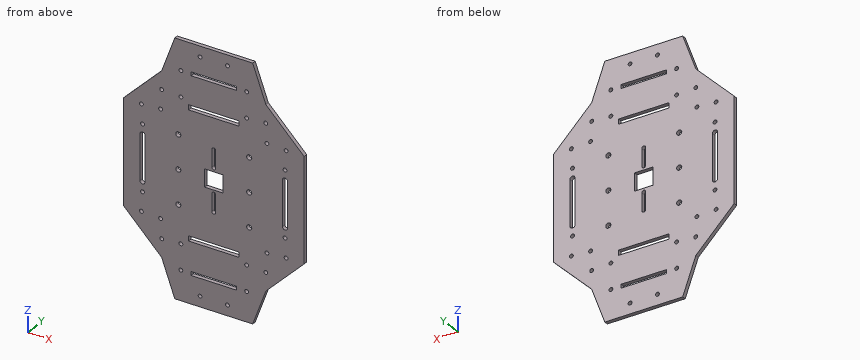
```python
from build123d import *

# Parameters (mm, degrees)
SKETCH_1_W                                 = 141.421356238
SKETCH_1_H                                 = 141.421356238
EXTRUDE_1_DEPTH                            = 3
CUT_EXTRUDE_1_DEPTH                        = 3
MIRROR_1_AT_THE_SECOND_PLANE_COPY_1_DEPTH  = 3
SKETCH_3_R                                 = 1.5
CUT_EXTRUDE_2_DEPTH                        = 3
MIRROR_2_AT_THE_SECOND_PLANE_COPY_1_SKET_R = 1.5
MIRROR_2_AT_THE_SECOND_PLANE_COPY_1_DEPTH  = 3
SKETCH_4_R                                 = 2
CUT_EXTRUDE_3_DEPTH                        = 3
SKETCH_5_R                                 = 1.5
CUT_EXTRUDE_4_DEPTH                        = 3
MIRROR_4_AT_THE_SECOND_PLANE_COPY_1_SKET_R = 1.5
MIRROR_4_AT_THE_SECOND_PLANE_COPY_1_DEPTH  = 3
SKETCH_6_R                                 = 1.5
CUT_EXTRUDE_5_DEPTH                        = 3
MIRROR_5_AT_THE_SECOND_PLANE_COPY_1_SKET_R = 1.5
MIRROR_5_AT_THE_SECOND_PLANE_COPY_1_DEPTH  = 3
CUT_EXTRUDE_6_DEPTH                        = 3
SKETCH_8_W                                 = 14.436516826
SKETCH_8_H                                 = 13.841494932
CUT_EXTRUDE_7_DEPTH                        = 3
CUT_EXTRUDE_8_DEPTH                        = 3
CUT_EXTRUDE_10_DEPTH                       = 3
EXTRUDE_2_DEPTH                            = 3
MIRROR_9_AT_THE_SECOND_PLANE_COPY_1_DEPTH  = 3
SKETCH_13_R                                = 1.5
CUT_EXTRUDE_11_DEPTH                       = 3
MIRROR_11_COPY_1_SKETCH_R                  = 1.5
MIRROR_11_COPY_1_DEPTH                     = 3


with BuildPart() as part:
    # 草图1 → 凸台-拉伸1 (new body)
    with BuildSketch(Plane(origin=(0, 0, 0), x_dir=(1, 0, 0), z_dir=(0, 1, 0))):
        Rectangle(SKETCH_1_W, SKETCH_1_H)
    extrude(amount=EXTRUDE_1_DEPTH)

    # 草图2 → 切除-拉伸1 (cut)
    with BuildSketch(Plane(origin=(0, 0, 0), x_dir=(1, 0, 0), z_dir=(0, 1, 0))):
        Polygon((-70.710678119, 70.710678119), (-40.710678119, 70.710678119), (-70.710678119, 40.710678119), align=None)
    cut_extrude_1 = extrude(amount=CUT_EXTRUDE_1_DEPTH, mode=Mode.SUBTRACT)

    # 镜向1: 切除-拉伸1 across plane
    add(cut_extrude_1.mirror(Plane(origin=(0, 0, 0), x_dir=(0, 0, 1), z_dir=(1, 0, 0))), mode=Mode.SUBTRACT)

    # 镜向1 at the second plane: 切除-拉伸1 across plane
    add(cut_extrude_1.mirror(Plane.XY), mode=Mode.SUBTRACT)

    # 镜向1 at the second plane copy 1 sket → 镜向1 at the second plane copy 1 (cut)
    with BuildSketch(Plane(origin=(0, 0, 0), x_dir=(-1, 0, 0), z_dir=(0, 1, 0))):
        Polygon((-70.710678119, 70.710678119), (-40.710678119, 70.710678119), (-70.710678119, 40.710678119), align=None)
    extrude(amount=MIRROR_1_AT_THE_SECOND_PLANE_COPY_1_DEPTH, mode=Mode.SUBTRACT)

    # 草图3 → 切除-拉伸2 (cut)
    with BuildSketch(Plane(origin=(0, 0, 0), x_dir=(1, 0, 0), z_dir=(0, 1, 0))):
        with Locations(Location((-56.568542495, 40.710678119, 0), (0, 0, 270))):
            Circle(SKETCH_3_R)
        with Locations(Location((-40.710678119, 56.568542495, 0), (0, 0, 270))):
            Circle(SKETCH_3_R)
        with Locations(Location((-41.568542495, 41.568542495, 0), (0, 0, 270))):
            Circle(SKETCH_3_R)
    cut_extrude_2 = extrude(amount=CUT_EXTRUDE_2_DEPTH, mode=Mode.SUBTRACT)

    # 镜向2: 切除-拉伸2 across plane
    add(cut_extrude_2.mirror(Plane.XY), mode=Mode.SUBTRACT)

    # 镜向2 at the second plane: 切除-拉伸2 across plane
    add(cut_extrude_2.mirror(Plane(origin=(0, 0, 0), x_dir=(0, 0, 1), z_dir=(1, 0, 0))), mode=Mode.SUBTRACT)

    # 镜向2 at the second plane copy 1 sket → 镜向2 at the second plane copy 1 (cut)
    with BuildSketch(Plane(origin=(0, 0, 0), x_dir=(-1, 0, 0), z_dir=(0, 1, 0))):
        with Locations(Location((-56.568542495, 40.710678119, 0), (0, 0, 270))):
            Circle(MIRROR_2_AT_THE_SECOND_PLANE_COPY_1_SKET_R)
        with Locations(Location((-40.710678119, 56.568542495, 0), (0, 0, 270))):
            Circle(MIRROR_2_AT_THE_SECOND_PLANE_COPY_1_SKET_R)
        with Locations(Location((-41.568542495, 41.568542495, 0), (0, 0, 270))):
            Circle(MIRROR_2_AT_THE_SECOND_PLANE_COPY_1_SKET_R)
    extrude(amount=MIRROR_2_AT_THE_SECOND_PLANE_COPY_1_DEPTH, mode=Mode.SUBTRACT)

    # 草图4 → 切除-拉伸3 (cut)
    with BuildSketch(Plane(origin=(0, 0, 0), x_dir=(1, 0, 0), z_dir=(0, 1, 0))):
        with Locations(Location((-27.710678119, 26.568542495, 0), (0, 0, 270))):
            Circle(SKETCH_4_R)
        with Locations(Location((-27.710678119, -26.568542495, 0), (0, 0, 270))):
            Circle(SKETCH_4_R)
        with Locations(Location((-27.710678119, 0, 0), (0, 0, 270))):
            Circle(SKETCH_4_R)
    cut_extrude_3 = extrude(amount=CUT_EXTRUDE_3_DEPTH, mode=Mode.SUBTRACT)

    # 镜向3: 切除-拉伸3 across plane
    add(cut_extrude_3.mirror(Plane(origin=(0, 0, 0), x_dir=(0, 0, 1), z_dir=(1, 0, 0))), mode=Mode.SUBTRACT)

    # 草图5 → 切除-拉伸4 (cut)
    with BuildSketch(Plane(origin=(0, 0, 0), x_dir=(1, 0, 0), z_dir=(0, 1, 0))):
        with Locations(Location((-55.710678119, 25.710678119, 0), (0, 0, 270))):
            Circle(SKETCH_5_R)
    cut_extrude_4 = extrude(amount=CUT_EXTRUDE_4_DEPTH, mode=Mode.SUBTRACT)

    # 镜向4: 切除-拉伸4 across plane
    add(cut_extrude_4.mirror(Plane(origin=(0, 0, 0), x_dir=(0, 0, 1), z_dir=(1, 0, 0))), mode=Mode.SUBTRACT)

    # 镜向4 at the second plane: 切除-拉伸4 across plane
    add(cut_extrude_4.mirror(Plane.XY), mode=Mode.SUBTRACT)

    # 镜向4 at the second plane copy 1 sket → 镜向4 at the second plane copy 1 (cut)
    with BuildSketch(Plane(origin=(0, 0, 0), x_dir=(-1, 0, 0), z_dir=(0, 1, 0))):
        with Locations(Location((-55.710678119, 25.710678119, 0), (0, 0, 270))):
            Circle(MIRROR_4_AT_THE_SECOND_PLANE_COPY_1_SKET_R)
    extrude(amount=MIRROR_4_AT_THE_SECOND_PLANE_COPY_1_DEPTH, mode=Mode.SUBTRACT)

    # 草图6 → 切除-拉伸5 (cut)
    with BuildSketch(Plane(origin=(0, 0, 0), x_dir=(1, 0, 0), z_dir=(0, 1, 0))):
        with Locations(Location((-25.710678119, 55.710678119, 0), (0, 0, 270))):
            Circle(SKETCH_6_R)
    cut_extrude_5 = extrude(amount=CUT_EXTRUDE_5_DEPTH, mode=Mode.SUBTRACT)

    # 镜向5: 切除-拉伸5 across plane
    add(cut_extrude_5.mirror(Plane.XY), mode=Mode.SUBTRACT)

    # 镜向5 at the second plane: 切除-拉伸5 across plane
    add(cut_extrude_5.mirror(Plane(origin=(0, 0, 0), x_dir=(0, 0, 1), z_dir=(1, 0, 0))), mode=Mode.SUBTRACT)

    # 镜向5 at the second plane copy 1 sket → 镜向5 at the second plane copy 1 (cut)
    with BuildSketch(Plane(origin=(0, 0, 0), x_dir=(-1, 0, 0), z_dir=(0, 1, 0))):
        with Locations(Location((-25.710678119, 55.710678119, 0), (0, 0, 270))):
            Circle(MIRROR_5_AT_THE_SECOND_PLANE_COPY_1_SKET_R)
    extrude(amount=MIRROR_5_AT_THE_SECOND_PLANE_COPY_1_DEPTH, mode=Mode.SUBTRACT)

    # 草图7 → 切除-拉伸6 (cut)
    with BuildSketch(Plane(origin=(0, 0, 0), x_dir=(1, 0, 0), z_dir=(0, 1, 0))):
        with BuildLine():
            Line((-53.710678119, 17.710678119), (-53.710678119, -17.710678119))
            ThreePointArc((-53.710678119, -17.710678119), (-55.710678119, -19.710678119), (-57.710678119, -17.710678119))
            Line((-57.710678119, -17.710678119), (-57.710678119, 17.710678119))
            ThreePointArc((-57.710678119, 17.710678119), (-55.710678119, 19.710678119), (-53.710678119, 17.710678119))
        make_face()
    cut_extrude_6 = extrude(amount=CUT_EXTRUDE_6_DEPTH, mode=Mode.SUBTRACT)

    # 镜向6: 切除-拉伸6 across plane
    add(cut_extrude_6.mirror(Plane(origin=(0, 0, 0), x_dir=(0, 0, 1), z_dir=(1, 0, 0))), mode=Mode.SUBTRACT)

    # 草图8 → 切除-拉伸7 (cut)
    with BuildSketch(Plane(origin=(0, 0, 0), x_dir=(1, 0, 0), z_dir=(0, 1, 0))):
        Rectangle(SKETCH_8_W, SKETCH_8_H)
    extrude(amount=CUT_EXTRUDE_7_DEPTH, mode=Mode.SUBTRACT)

    # 草图9 → 切除-拉伸8 (cut)
    with BuildSketch(Plane(origin=(0, 0, 0), x_dir=(1, 0, 0), z_dir=(0, 1, 0))):
        with BuildLine():
            Line((1.5, -9.920747466), (1.5, -23.568542495))
            ThreePointArc((1.5, -23.568542495), (0, -25.068542495), (-1.5, -23.568542495))
            Line((-1.5, -23.568542495), (-1.5, -9.920747466))
            ThreePointArc((-1.5, -9.920747466), (0, -8.420747466), (1.5, -9.920747466))
        make_face()
    cut_extrude_8 = extrude(amount=CUT_EXTRUDE_8_DEPTH, mode=Mode.SUBTRACT)

    # 镜向7: 切除-拉伸8 across plane
    add(cut_extrude_8.mirror(Plane.XY), mode=Mode.SUBTRACT)

    # 草图10 → 切除-拉伸10 (cut)
    with BuildSketch(Plane(origin=(0, 0, 0), x_dir=(1, 0, 0), z_dir=(0, 1, 0))):
        Polygon((-19.710678119, 51.710678119), (-19.710678119, 51.490395466), (-19.710678119, 47.710678119), (19.710678119, 47.710678119), (19.710678119, 51.710678119), align=None)
    cut_extrude_10 = extrude(amount=CUT_EXTRUDE_10_DEPTH, mode=Mode.SUBTRACT)

    # 镜向8: 切除-拉伸10 across plane
    add(cut_extrude_10.mirror(Plane.XY), mode=Mode.SUBTRACT)

    # 草图11 → 凸台-拉伸2 (add)
    with BuildSketch(Plane(origin=(0, 3, 0), x_dir=(1, 0, 0), z_dir=(0, 1, 0))):
        Polygon((-40.710678119, 70.710678119), (-30.450073819, 98.901456742), (30.450073819, 98.901456742), (40.710678119, 70.710678119), align=None)
    extrude_2 = extrude(amount=-EXTRUDE_2_DEPTH)

    # 镜向9: 凸台-拉伸2 across plane
    add(extrude_2.mirror(Plane(origin=(0, 0, 0), x_dir=(0, 0, 1), z_dir=(1, 0, 0))))

    # 镜向9 at the second plane: 凸台-拉伸2 across plane
    add(extrude_2.mirror(Plane.XY))

    # 镜向9 at the second plane copy 1 sket → 镜向9 at the second plane copy 1 (add)
    with BuildSketch(Plane(origin=(0, 3, 0), x_dir=(-1, 0, 0), z_dir=(0, 1, 0))):
        Polygon((-40.710678119, 70.710678119), (-30.450073819, 98.901456742), (30.450073819, 98.901456742), (40.710678119, 70.710678119), align=None)
    extrude(amount=-MIRROR_9_AT_THE_SECOND_PLANE_COPY_1_DEPTH)

    # 草图13 → 切除-拉伸11 (cut)
    with BuildSketch(Plane.XZ):
        with Locations(Location((-25.710678119, 75.710678119, 0), (0, 0, 270))):
            Circle(SKETCH_13_R)
        with Locations(Location((-10.710678119, 90.710678119, 0), (0, 0, 270))):
            Circle(SKETCH_13_R)
        Polygon((-17.710678119, 75.710678119), (-17.710678119, 77.210678119), (0, 77.210678119), (0, 74.210678119), (-17.710678119, 74.210678119), align=None)
    cut_extrude_11 = extrude(amount=-CUT_EXTRUDE_11_DEPTH, mode=Mode.SUBTRACT)

    # 镜向10: 切除-拉伸11 across plane
    add(cut_extrude_11.mirror(Plane(origin=(0, 0, 0), x_dir=(0, 0, 1), z_dir=(1, 0, 0))), mode=Mode.SUBTRACT)

    # 镜向11: 切除-拉伸11 across plane
    add(cut_extrude_11.mirror(Plane.XY), mode=Mode.SUBTRACT)

    # 镜向11 copy 1 sketch → 镜向11 copy 1 (cut)
    with BuildSketch(Plane(origin=(0, 0, 0), x_dir=(-1, 0, 0), z_dir=(0, -1, 0))):
        with Locations(Location((-25.710678119, 75.710678119, 0), (0, 0, 270))):
            Circle(MIRROR_11_COPY_1_SKETCH_R)
        with Locations(Location((-10.710678119, 90.710678119, 0), (0, 0, 270))):
            Circle(MIRROR_11_COPY_1_SKETCH_R)
        Polygon((-17.710678119, 75.710678119), (-17.710678119, 77.210678119), (0, 77.210678119), (0, 74.210678119), (-17.710678119, 74.210678119), align=None)
    extrude(amount=-MIRROR_11_COPY_1_DEPTH, mode=Mode.SUBTRACT)


solid = part.part
```
Could you check a few things on this model? Use its own coordinates, in mm. Coordinates: 2 decimals unless noted, no trailing zeros. Loops run counter-clockwise (first coordinate to the right, second up) from the corner with the lowest first, then second, coordinate; pieces in that order, holes last.
1) Will these pins go through, and if not, where does the flat tip stop? pin 1 Ø1 at (y, z) = (1.5, -70) entering from +X; pin 2 Ø4 at (x, z) = (-10.71, -90.71) entering from -Y.
Reported:
pin 1: stops at x = 41.92
pin 2: stops at y = 0
2) Imagine slicing it at A-A (z = 0). List the corners of the cut face in (x, y) for me, and give its area (3 significant figures).
Reported:
outline: (-70.71, 0) - (-57.71, 0) - (-57.71, 3) - (-70.71, 3) - close; (-53.71, 0) - (-29.71, 0) - (-29.71, 3) - (-53.71, 3) - close; (-25.71, 0) - (-7.22, 0) - (-7.22, 3) - (-25.71, 3) - close; (7.22, 0) - (25.71, 0) - (25.71, 3) - (7.22, 3) - close; (29.71, 0) - (53.71, 0) - (53.71, 3) - (29.71, 3) - close; (57.71, 0) - (70.71, 0) - (70.71, 3) - (57.71, 3) - close
area: 333 mm2
3) Please list where these lines run through material, in increasing order: line 1 along Z through (x, y) = (17.5, 0.75); line 2 along X through (y, z) = (2.55, 13.5); line 3 along Z through (x, y) = (6.5, 1.55).
Reported:
line 1: z = -98.9 to -77.21, -74.21 to -51.71, -47.71 to 47.71, 51.71 to 74.21, 77.21 to 98.9
line 2: x = -70.71 to -57.71, -53.71 to -1.5, 1.5 to 53.71, 57.71 to 70.71
line 3: z = -98.9 to -77.21, -74.21 to -51.71, -47.71 to -6.92, 6.92 to 47.71, 51.71 to 74.21, 77.21 to 98.9
4) Imagine slicing it at C-C (x = 45.5). List the corners of the cut face in (y, z) for me.
Reported:
outline: (0, -65.92) - (3, -65.92) - (3, 65.92) - (0, 65.92) - close
5) Imagine slicing it at B-B (y = 1.25). State how many separate pieces and enclosed holes the cut face has, and give its area (3 significant figures).
Reported:
separate pieces: 1
enclosed holes: 43
area: 20,800 mm2
